Here's how the part is built. I have some questions about the finished solid (model axes, mm). A direction names the side the tool comes from. Coordinates: 2 decimals unless noted, no trailing zeros. Order: outer loops, then holes, each group sorted by start corner. A loop starts at its lowest first (then second) coordinate and runs counter-clockwise, first axis right, second up. Notation, with made-up numbers: (-20.5, -37) - (13.5, -37) arc R34 cw to (13.5, -4) - close; hole circle Ø1 at (33.25, 56). An arc over 180 degrees is marked (long way). Answer in a Markdown table with one row per item. Add a question column.
Item 1: If I drill on line 1 along X through (y, z) = (20, -7); line 2 along Y through (x, z) = (55, -13.5); line 3 along X through (y, z) = (14, -16.5), over which ranges is the centre line in solid material (lowest first)? Write a range as from..to.
Item 2: Will these pins go through, and if not, where does the flat tip stop? pin 1 Ø12 at (x, y) = (28, 23) entering from -Z; pin 2 Ø1 at (x, y) = (52.5, 18) entering from +Z; pin 3 Ø0.8 at (x, z) = (5, -25.5) entering from +Y.
Item 3: On a 3-axis mill with a long thin cutter (end or side, diameter ignored), from which of +Z, -Z, +X, -X, +Y, -Y can I reach the whole of each face in a straight line? I mean faces 4 (the flat face through (60, 12, -16)), 5 (the cylindrical face through (52.226, 20.163, -9.93)), 6 (the cylindrical face through (1.4, 8.62, -21.63)). Say none if no direction works.
Item 4: Thinking about a two-plate mould opening in Y: for faces 1 (the flat face through (30, 2, -40)), 2 (the flat face through (56.6, 22.3, -15)), 3 (the cylindrical face through (51.77, 12.129, -22.518)), which applies, +Y half, -Y half, draft (parallel to the pull), parting line (faces both ways), or undercut?
Item 5: I want a section at A-A (x = 20). Please give me the cut outline in (y, z), plus the area to 3 significant figures.
Item 6: I want a section at B-B (z = -3). Please give me the cut outline in (x, y), plus the area to 3 significant figures.
```python
from build123d import *

# Parameters (mm, degrees)
SKETCH1_W            = 60
SKETCH1_H            = 40
BOSS_EXTRUDE1_DEPTH  = 5
SKETCH2_W            = 9.75
SKETCH2_H            = 10
BOSS_EXTRUDE2_DEPTH  = 26
BOSS_EXTRUDE3_DEPTH  = 9.75
CUT_EXTRUDE1_DEPTH   = 36
SKETCH5_W            = 10
SKETCH5_H            = 5
BOSS_EXTRUDE4_DEPTH  = 40.5
WIRE_CUT_OUT_DEPTH   = 36.0000001
WASHER_CUT_OUT_DEPTH = 25
FILLET1_R            = 1


with BuildPart() as part:
    # Sketch1 → Boss-Extrude1 (new body)
    with BuildSketch(Plane(origin=(0, 0, 0), x_dir=(1, 0, 0), z_dir=(0, 1, 0))):
        with Locations((30, 20)):
            Rectangle(SKETCH1_W, SKETCH1_H)
    extrude(amount=BOSS_EXTRUDE1_DEPTH)

    # Sketch2 → Boss-Extrude2 (add)
    with BuildSketch(Plane(origin=(0, 5, 0), x_dir=(1, 0, 0), z_dir=(0, 1, 0))):
        with Locations((4.875, 10)):
            Rectangle(SKETCH2_W, SKETCH2_H)
        with Locations((55.125, 10)):
            Rectangle(SKETCH2_W, SKETCH2_H)
    extrude(amount=BOSS_EXTRUDE2_DEPTH)

    # Sketch3 → Boss-Extrude3 (add)
    with BuildSketch(Plane.ZY):
        with BuildLine():
            Line((-15, 30), (-15, 5))
            Line((-15, 5), (-40, 5))
            ThreePointArc((-40, 5), (-22.32233047, 12.32233047), (-15, 30))
        make_face()
    boss_extrude3 = extrude(amount=-BOSS_EXTRUDE3_DEPTH)

    # Mirror2: Boss-Extrude3 across plane
    add(boss_extrude3.mirror(Plane(origin=(30, 0, 0), x_dir=(0, 0, 1), z_dir=(1, 0, 0))))

    # Sketch4 → Cut-Extrude1 (cut, through all)
    with BuildSketch(Plane.XY.offset(-5)):
        with BuildLine():
            Line((4.5, 22.388), (5.5, 22.388))
            ThreePointArc((5.5, 22.388), (7.775, 20.113), (5.5, 17.838))
            Line((5.5, 17.838), (4.5, 17.838))
            ThreePointArc((4.5, 17.838), (2.225, 20.113), (4.5, 22.388))
        make_face()
        with BuildLine():
            Line((4.5, 11.952), (5.5, 11.952))
            ThreePointArc((5.5, 11.952), (7.775, 9.677), (5.5, 7.402))
            Line((5.5, 7.402), (4.5, 7.402))
            ThreePointArc((4.5, 7.402), (2.225, 9.677), (4.5, 11.952))
        make_face()
        with BuildLine():
            Line((55.5, 11.952), (54.5, 11.952))
            ThreePointArc((54.5, 11.952), (52.225, 9.677), (54.5, 7.402))
            Line((54.5, 7.402), (55.5, 7.402))
            ThreePointArc((55.5, 7.402), (57.775, 9.677), (55.5, 11.952))
        make_face()
        with BuildLine():
            Line((55.5, 22.388), (54.5, 22.388))
            ThreePointArc((54.5, 22.388), (52.225, 20.113), (54.5, 17.838))
            Line((54.5, 17.838), (55.5, 17.838))
            ThreePointArc((55.5, 17.838), (57.775, 20.113), (55.5, 22.388))
        make_face()
    extrude(amount=-CUT_EXTRUDE1_DEPTH, mode=Mode.SUBTRACT)

    # Sketch5 → Boss-Extrude4 (add)
    with BuildSketch(Plane(origin=(9.75, 0, 0), x_dir=(0, 0, -1), z_dir=(1, 0, 0))):
        with Locations((10, 28.5)):
            Rectangle(SKETCH5_W, SKETCH5_H)
    extrude(amount=BOSS_EXTRUDE4_DEPTH)

    # Sketch6 → Wire_Cut_Out (cut, through all)
    with BuildSketch(Plane.XY.offset(-5)):
        with BuildLine():
            Line((5.5, 17.838), (5, 17.838))
            Line((5, 17.838), (5, 11.952))
            Line((5, 11.952), (5.5, 11.952))
            ThreePointArc((5.5, 11.952), (6.559361256, 11.690300457), (7.375, 10.965409873))
            Line((7.375, 10.965409873), (9.75, 10.965409873))
            Line((9.75, 10.965409873), (9.75, 18.824590127))
            Line((9.75, 18.824590127), (7.375, 18.824590127))
            ThreePointArc((7.375, 18.824590127), (6.559361256, 18.099699543), (5.5, 17.838))
        make_face()
        with BuildLine():
            Line((5, 18.824590127), (5, 17.838))
            Line((5, 17.838), (5.5, 17.838))
            ThreePointArc((5.5, 17.838), (6.559361256, 18.099699543), (7.375, 18.824590127))
            Line((7.375, 18.824590127), (5, 18.824590127))
        make_face()
        with BuildLine():
            Line((5.5, 11.952), (5, 11.952))
            Line((5, 11.952), (5, 10.965409873))
            Line((5, 10.965409873), (7.375, 10.965409873))
            ThreePointArc((7.375, 10.965409873), (6.559361256, 11.690300457), (5.5, 11.952))
        make_face()
    extrude(amount=-WIRE_CUT_OUT_DEPTH, mode=Mode.SUBTRACT)

    # Sketch8 → Washer_Cut_Out (cut)
    with BuildSketch(Plane(origin=(0, 0, -40), x_dir=(-1, 0, 0), z_dir=(0, 0, -1))):
        with BuildLine():
            Line((-55.5, 23.388), (-54.5, 23.388))
            ThreePointArc((-54.5, 23.388), (-51.225, 20.113), (-54.5, 16.838))
            Line((-54.5, 16.838), (-55.5, 16.838))
            ThreePointArc((-55.5, 16.838), (-58.775, 20.113), (-55.5, 23.388))
        make_face()
        with BuildLine():
            Line((-55.5, 12.952), (-54.5, 12.952))
            ThreePointArc((-54.5, 12.952), (-51.225, 9.677), (-54.5, 6.402))
            Line((-54.5, 6.402), (-55.5, 6.402))
            ThreePointArc((-55.5, 6.402), (-58.775, 9.677), (-55.5, 12.952))
        make_face()
        with BuildLine():
            Line((-5.5, 23.388), (-4.5, 23.388))
            ThreePointArc((-4.5, 23.388), (-1.225, 20.113), (-4.5, 16.838))
            Line((-4.5, 16.838), (-5.5, 16.838))
            ThreePointArc((-5.5, 16.838), (-8.775, 20.113), (-5.5, 23.388))
        make_face()
        with BuildLine():
            Line((-5.5, 12.952), (-4.5, 12.952))
            ThreePointArc((-4.5, 12.952), (-1.225, 9.677), (-4.5, 6.402))
            Line((-4.5, 6.402), (-5.5, 6.402))
            ThreePointArc((-5.5, 6.402), (-8.775, 9.677), (-5.5, 12.952))
        make_face()
    extrude(amount=-WASHER_CUT_OUT_DEPTH, mode=Mode.SUBTRACT)

    # Fillet1
    fillet1_edges = [part.edges().sort_by_distance(p)[0] for p in [
        (60, 5, -2.5),
        (0, 5, -2.5),
        (50.25, 15.5, -5),
        (9.75, 22.412295064, -5),
        (30, 26, -15),
        (30, 26, -5),
        (0, 30.5, -15),
        (0, 18, -5),
        (9.75, 6.538704712, -31.364745319),
        (9.75, 7.982704936, -5),
        (0, 31, -10),
        (30, 31, -5),
        (60, 18, -5),
        (60, 30.5, -15),
        (60, 31, -10),
        (0, 12.32233047, -22.32233047),
        (60, 12.32233047, -22.32233047),
        (60, 0, -20),
        (30, 0, 0),
        (0, 0, -20),
        (0, 2.5, -40),
        (60, 2.5, -40),
        (60, 2.5, 0),
        (0, 2.5, 0),
        (30, 5, 0),
    ]]
    fillet(fillet1_edges, radius=FILLET1_R)


solid = part.part
```
Values follow:
| question | item | result |
|---|---|---|
| 1 | line 1 | x = 0..2.23, 7.77..9.75, 50.25..52.23, 57.77..60 |
| 1 | line 2 | y = 0..7.4, 11.95..17.84, 22.39..31 |
| 1 | line 3 | x = 0..5, 50.25..60 |
| 2 | pin 1 | stops at z = -15 |
| 2 | pin 2 | stops at z = -5 |
| 2 | pin 3 | stops at y = 6.4 |
| 3 | face 4 | +Z, -Z, +X, +Y, -Y |
| 3 | face 5 | +Z, -Z |
| 3 | face 6 | -Z |
| 4 | face 1 | draft |
| 4 | face 2 | undercut |
| 4 | face 3 | +Y half |
| 5 | outline | (0, -40) - (5, -40) - (5, -1) arc R1 ccw to (4, 0) - (1, 0) arc R1 ccw to (0, -1) - close; (26, -14) arc R1 ccw to (27, -15) - (31, -15) - (31, -6) arc R1 ccw to (30, -5) - (27, -5) arc R1 ccw to (26, -6) - close |
| 5 | area | 249 mm^2 |
| 6 | outline | (0, 1) arc R1 ccw to (1, 0) - (59, 0) arc R1 ccw to (60, 1) - (60, 4) arc R1 ccw to (59, 5) - (1, 5) arc R1 ccw to (0, 4) - close |
| 6 | area | 299 mm^2 |
